from build123d import *

# Parameters (mm, degrees)
BOX001_W      = 6
BOX001_H      = 17
BOX001_DEPTH  = 5
BOX_W         = 11.5
BOX_H         = 31.5
BOX_DEPTH     = 40
EXTRUDE_DEPTH = 41.5


with BuildPart() as cube001:
    # Box001 → Box001 (new body)
    with BuildSketch(Plane(origin=(-33.030017, -29.25, 15.266888), x_dir=(1, 0, 0), z_dir=(0, 0, 1))):
        with Locations((3, 8.5)):
            Rectangle(BOX001_W, BOX001_H)
    extrude(amount=BOX001_DEPTH)


with BuildPart() as cube:
    # Box → Box (new body)
    with BuildSketch(Plane(origin=(-36.280017, -36.5, 20.266888), x_dir=(1, 0, 0), z_dir=(0, 0, 1))):
        with Locations((5.75, 15.75)):
            Rectangle(BOX_W, BOX_H)
    extrude(amount=BOX_DEPTH)


with BuildPart() as cut001:
    # Sketch → Extrude (new body)
    with BuildSketch(Plane.XZ):
        Polygon((-13.050017, 40.266888), (-9.280017, 40.266888), (-9.280017, 60.266888), (-20.280017, 60.266888), (-40.780017, 60.266888), (-40.780017, 15.266888), (-19.280017, 15.266888), (-19.280017, 56.266888), (-12.050017, 56.266888), (-13.050017, 42.266888), align=None)
    extrude(amount=EXTRUDE_DEPTH)

    # Cut: cut Cube
    add(cube.part, mode=Mode.SUBTRACT)

    # Cut001: cut Cube001
    add(cube001.part, mode=Mode.SUBTRACT)


solid = cut001.part
Design review of the part built by this model. Coordinates are the model's own, in mm. A direction names the side the tool comes from. Round coordinates to 2 decimals unless told otherwise and drop trailing zeros. Order: outer loops, then holes, each group sorted by start corner. A loop starts at its lowest first (then second) coordinate and runs counter-clockwise, first axis right, second up. Notation, with made-up numbers: M -24.5,-3.75 L 12.5,-3.75 A14 ccw 12.5,4.25 Z; hole C -21,-22.75 d2. An arc over 180 degrees is marked long. Answer as CSV lines item,"result". Start each with the question number.
1) Tool access review of faces 1 (the face through (-31, -5, 40)), 2 (the face through (-30, -12.25, 18)), 3 (the face through (-11, -20, 40.267)), 4 (the face through (-13.05, -20, 41)): name each direction out of +Z, -Z, +X, -X, +Y, -Y from which nothing blocks a thin tool from reaching the whole face with its end or side.
2) Add section A-A (z = 41.5). Give the boundary of the cut face in (x, y), then the cut area to 3 significant figures.
3) For pin 1 Ø1 at (x, y) = (-25.5, -26.5) entering from +Z; pin 2 Ø1.5 at (y, z) = (-23.5, 17.5) entering from +X; pin 3 Ø4 at (x, y) = (-12, -17) entering from -Z, all flat-tipped, find the tip position at first contact; note any pin that passes through.
4) Add section D-D (z = 30.5). Give the boundary of the cut face in (x, y).
5) The part is to be moulded in two halves that separate along X. For faces 5 (the face through (-29, 0, 38)), 6 (the face through (-30, -29.25, 18)), 7 (the face through (-40.78, -20, 38)), 8 (the face through (-24.78, -21, 40)), say which applies: +X half, -X half, draft (parallel to the pull), parting line (faces both ways), or undercut.
6) Add section B-B (y = -22.5). Give the boundary of the cut face in (x, z), then the cut area to 3 significant figures.
7) Add section C-C (y = -11). Give the boundary of the cut face in (x, z), then the cut area to 3 significant figures.
8) Wall thickness on line 1 along Y through (x, z) = (-27.5, 41.5); line 2 along X through (y, z) = (-36, 24.5); line 3 along X through (y, z) = (-33.5, 58): over which ranges is each line inside the solid? List them lowest first. Write a range as [from, to].
Resolved:
1,face 1,"+Z"
1,face 2,"+Z, -Z"
1,face 3,"-Z, +X, +Y, -Y"
1,face 4,"-Z, +Y, -Y"
2,outline,"M -40.78,-41.5 L -19.28,-41.5 L -19.28,0 L -40.78,0 Z; M -13.05,-41.5 L -9.28,-41.5 L -9.28,0 L -13.05,0 Z; hole M -36.28,-36.5 L -24.78,-36.5 L -24.78,-5 L -36.28,-5 Z"
2,area,"686 mm^2"
3,pin 1,"z = 20.27"
3,pin 2,"x = -19.28"
3,pin 3,"z = 40.27"
4,outline,"M -40.78,-41.5 L -19.28,-41.5 L -19.28,0 L -40.78,0 Z; hole M -36.28,-36.5 L -24.78,-36.5 L -24.78,-5 L -36.28,-5 Z"
5,face 5,"draft"
5,face 6,"undercut"
5,face 7,"-X half"
5,face 8,"undercut"
6,outline,"M -40.78,15.27 L -33.03,15.27 L -33.03,20.27 L -36.28,20.27 L -36.28,60.27 L -40.78,60.27 Z; M -27.03,15.27 L -19.28,15.27 L -19.28,56.27 L -12.05,56.27 L -13.05,42.27 L -13.05,40.27 L -9.28,40.27 L -9.28,60.27 L -24.78,60.27 L -24.78,20.27 L -27.03,20.27 Z"
6,area,"571 mm^2"
7,outline,"M -40.78,15.27 L -19.28,15.27 L -19.28,56.27 L -12.05,56.27 L -13.05,42.27 L -13.05,40.27 L -9.28,40.27 L -9.28,60.27 L -24.78,60.27 L -24.78,20.27 L -36.28,20.27 L -36.28,60.27 L -40.78,60.27 Z"
7,area,"601 mm^2"
8,line 1,"[-41.5, -36.5], [-5, 0]"
8,line 2,"[-40.78, -36.28], [-24.78, -19.28]"
8,line 3,"[-40.78, -36.28], [-24.78, -9.28]"
